from build123d import *

# Parameters (mm, degrees)
F0_R     = 1.5
F1_DEPTH = 5


with BuildPart() as f1:
    # F0 (on Front) → F1 (new body)
    with BuildSketch(Plane.XZ):
        with BuildLine():
            ThreePointArc((4.885955, -1.061812), (4.971407, -0.533959), (5, 0))
            ThreePointArc((5, 0), (4.971407, 0.533959), (4.885955, 1.061812))
            ThreePointArc((4.885955, 1.061812), (4.755283, 1.545085), (4.576938, 2.012868))
            ThreePointArc((4.576938, 2.012868), (4.045085, 2.938926), (3.328703, 3.730916))
            ThreePointArc((3.328703, 3.730916), (2.938926, 4.045085), (2.519686, 4.318701))
            ThreePointArc((2.519686, 4.318701), (1.545085, 4.755283), (0.5, 4.974937))
            ThreePointArc((0.5, 4.974937), (0, 5), (-0.5, 4.974937))
            ThreePointArc((-0.5, 4.974937), (-1.545085, 4.755283), (-2.519686, 4.318701))
            ThreePointArc((-2.519686, 4.318701), (-2.938926, 4.045085), (-3.328703, 3.730916))
            ThreePointArc((-3.328703, 3.730916), (-4.045085, 2.938926), (-4.576938, 2.012868))
            ThreePointArc((-4.576938, 2.012868), (-4.755283, 1.545085), (-4.885955, 1.061812))
            ThreePointArc((-4.885955, 1.061812), (-5, 0), (-4.885955, -1.061812))
            ThreePointArc((-4.885955, -1.061812), (-4.755283, -1.545085), (-4.576938, -2.012868))
            ThreePointArc((-4.576938, -2.012868), (-4.045085, -2.938926), (-3.328703, -3.730916))
            ThreePointArc((-3.328703, -3.730916), (-2.938926, -4.045085), (-2.519686, -4.318701))
            ThreePointArc((-2.519686, -4.318701), (-1.545085, -4.755283), (-0.5, -4.974937))
            ThreePointArc((-0.5, -4.974937), (0, -5), (0.5, -4.974937))
            ThreePointArc((0.5, -4.974937), (1.545085, -4.755283), (2.519686, -4.318701))
            ThreePointArc((2.519686, -4.318701), (2.938926, -4.045085), (3.328703, -3.730916))
            ThreePointArc((3.328703, -3.730916), (4.045085, -2.938926), (4.576938, -2.012868))
            ThreePointArc((4.576938, -2.012868), (4.755283, -1.545085), (4.885955, -1.061812))
        make_face()
        Circle(F0_R, mode=Mode.SUBTRACT)
        with BuildLine():
            ThreePointArc((4.576938, 2.012868), (4.755283, 1.545085), (4.885955, 1.061812))
            Line((4.885955, 1.061812), (6.336376, 1.533082))
            Line((6.336376, 1.533082), (6.027359, 2.484139))
            Line((6.027359, 2.484139), (4.576938, 2.012868))
        make_face()
        with BuildLine():
            Line((6.336376, -1.533082), (4.885955, -1.061812))
            ThreePointArc((4.885955, -1.061812), (4.755283, -1.545085), (4.576938, -2.012868))
            Line((4.576938, -2.012868), (6.027359, -2.484139))
            Line((6.027359, -2.484139), (6.336376, -1.533082))
        make_face()
        with BuildLine():
            ThreePointArc((2.519686, 4.318701), (2.938926, 4.045085), (3.328703, 3.730916))
            Line((3.328703, 3.730916), (4.225113, 4.964718))
            Line((4.225113, 4.964718), (3.416096, 5.552503))
            Line((3.416096, 5.552503), (2.519686, 4.318701))
        make_face()
        with BuildLine():
            Line((4.225113, -4.964718), (3.328703, -3.730916))
            ThreePointArc((3.328703, -3.730916), (2.938926, -4.045085), (2.519686, -4.318701))
            Line((2.519686, -4.318701), (3.416096, -5.552503))
            Line((3.416096, -5.552503), (4.225113, -4.964718))
        make_face()
        with BuildLine():
            ThreePointArc((-0.5, 4.974937), (0, 5), (0.5, 4.974937))
            Line((0.5, 4.974937), (0.5, 6.5))
            Line((0.5, 6.5), (-0.5, 6.5))
            Line((-0.5, 6.5), (-0.5, 4.974937))
        make_face()
        with BuildLine():
            Line((0.5, -6.5), (0.5, -4.974937))
            ThreePointArc((0.5, -4.974937), (0, -5), (-0.5, -4.974937))
            Line((-0.5, -4.974937), (-0.5, -6.5))
            Line((-0.5, -6.5), (0.5, -6.5))
        make_face()
        with BuildLine():
            ThreePointArc((-3.328703, 3.730916), (-2.938926, 4.045085), (-2.519686, 4.318701))
            Line((-2.519686, 4.318701), (-3.416096, 5.552503))
            Line((-3.416096, 5.552503), (-4.225113, 4.964718))
            Line((-4.225113, 4.964718), (-3.328703, 3.730916))
        make_face()
        with BuildLine():
            Line((-3.416096, -5.552503), (-2.519686, -4.318701))
            ThreePointArc((-2.519686, -4.318701), (-2.938926, -4.045085), (-3.328703, -3.730916))
            Line((-3.328703, -3.730916), (-4.225113, -4.964718))
            Line((-4.225113, -4.964718), (-3.416096, -5.552503))
        make_face()
        with BuildLine():
            ThreePointArc((-4.885955, 1.061812), (-4.755283, 1.545085), (-4.576938, 2.012868))
            Line((-4.576938, 2.012868), (-6.027359, 2.484139))
            Line((-6.027359, 2.484139), (-6.336376, 1.533082))
            Line((-6.336376, 1.533082), (-4.885955, 1.061812))
        make_face()
        with BuildLine():
            Line((-6.027359, -2.484139), (-4.576938, -2.012868))
            ThreePointArc((-4.576938, -2.012868), (-4.755283, -1.545085), (-4.885955, -1.061812))
            Line((-4.885955, -1.061812), (-6.336376, -1.533082))
            Line((-6.336376, -1.533082), (-6.027359, -2.484139))
        make_face()
    extrude(amount=F1_DEPTH)


solid = f1.part
Part model, mm, in its own coordinate system. A direction names the side the tool comes from. Give positions to 0.01 mm unless a question says otherwise; leave off trailing zeros. Loops run counter-clockwise (first coordinate to the right, second up) from the corner with the lowest first, then second, coordinate; pieces in that order, holes last. Notation, with made-up numbers: M -11,3 L 3,3 A22 cw 3,27 Z; hole C -1,87 d1. An arc over 180 degrees is marked long. Put each result on its own line as item: value. Start each with the question number.
1) Saw through at C-C (x = 3.75). List the corners of the cut face in (y, z).
2) Saw through at B-B (z = 2.25). List the corners of the cut face in (x, y).
3) Flat gauge pins, fed straight in: pin 1 (0.5 mm diameter, centred on y = -1.5, z = 6, fed in from -X); pin 2 (1.5 mm diameter, centred on x = -1.5, y = -4.5, fed in from +Z); pin 3 (1 mm diameter, centred on x = -5, y = -0.5, fed in from -Z); pin 4 (1.5 mm diameter, centred on y = -2.5, z = 1.5, fed in from -X). Where does each tip first touch, or does it go through?
4) Pull direction X, two halves, no side cores. Call faces 4 (the flat face through (6.18, -2.46, -2.02)), 5 (the flat face through (0, -5, 2)), 6 (the flat face through (-5.31, -2.46, -2.25)): +X half, -X half, draft (parallel to the pull), parting line (faces both ways), or undercut.
5) Saw through at D-D (z = -3). List the corners of the cut face in (x, y), then the cut area to 3 significant figures.
6) Probe probe 1 along Z at (x, y) = (0, -1.45); probe 2 along Z at (x, y) = (4, -2.15); probe 3 along Z at (x, y) = (2.25, -2.4). List the from-to ranges inside material, lowest first.
7) Saw through at A-A (x = 0). List the corners of the cut face in (y, z), then the cut area to 3 significant figures.
8) 3-axis set-ups, long thin cutter, end or side, ignore diameter. For faces 1 (the flat face through (-5.601, -2.465, -1.294)), 2 (the flat face through (-2.962, -2.465, 4.927)), 3 (the flat face through (5.601, -2.465, 1.294)): which of +Z, -Z, +X, -X, +Y, -Y reach the whole face in a straight line?
Numbers:
1. outline: M -5,-5.31 L 0,-5.31 L 0,-4.31 L -5,-4.31 Z; M -5,-3.31 L 0,-3.31 L 0,3.31 L -5,3.31 Z; M -5,4.31 L 0,4.31 L 0,5.31 L -5,5.31 Z
2. outline: M -6.1,-5 L -5.31,-5 L -5.31,0 L -6.1,0 Z; M -4.47,-5 L 4.47,-5 L 4.47,0 L -4.47,0 Z; M 5.31,-5 L 6.1,-5 L 6.1,0 L 5.31,0 Z
3. pin 1: x = -0.5
3. pin 2: z = 4.94
3. pin 3: z = -2.31
3. pin 4: x = -6.34
4. face 4: +X half
4. face 5: draft
4. face 6: undercut
5. outline: M -4,-5 L 4,-5 L 4,0 L -4,0 Z
5. area: 40.0 mm^2
6. probe 1: -6.5 to -1.5, 1.5 to 6.5
6. probe 2: -5.13 to -4.65, -3 to 3, 4.65 to 5.13
6. probe 3: -4.47 to 4.47
7. outline: M -5,-6.5 L 0,-6.5 L 0,-1.5 L -5,-1.5 Z; M -5,1.5 L 0,1.5 L 0,6.5 L -5,6.5 Z
7. area: 50.0 mm^2
8. face 1: -X, +Y, -Y
8. face 2: +Z, +Y, -Y
8. face 3: +X, +Y, -Y
